Check sheet for the drawn part. Datum: minimum x, y, z corner. Units: mm. A direction names the side the tool comes from. Round coordinates to 2 decimals unless told otherwise and drop trailing zeros. Loops run counter-clockwise (first coordinate to the right, second up) from the corner with the lowest first, then second, coordinate; pieces in that order, holes last. Notation, with made-up numbers: (-26, -35.75) -> (10, -35.75) arc R4 cw to (10, -31.75) -> close; hole circle Ø1 at (43.25, 64.25). An arc over 180 degrees is marked (long way). Use CSV: the item, a comma, the result in double quotes. Start each with the question number.
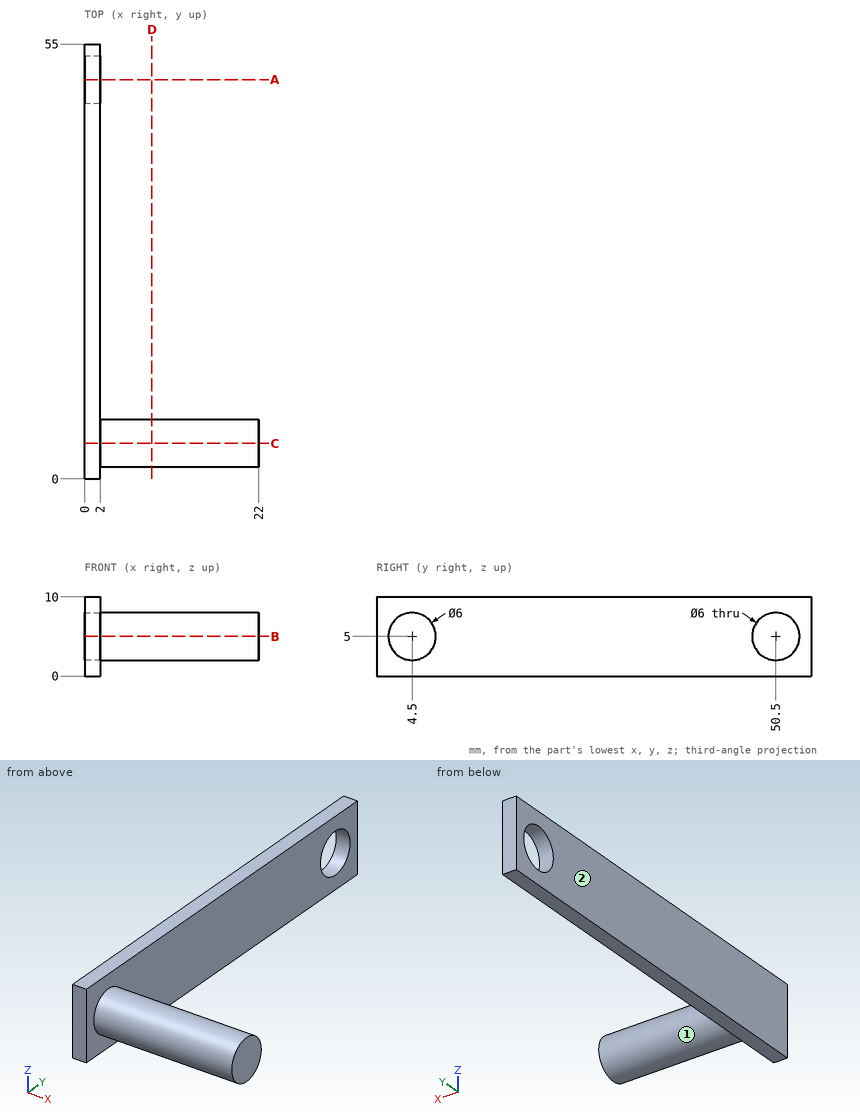
Q1. Cross-section at C-C (y = 4.5). Record the boundary of the cut face in (x, z), and give its area (3 significant figures).
Q2. Depth check by flat-ended pin: pin 1 Ø1 at (y, z) = (47, 6.5) entering from +X; pin 2 Ø4 at (y, z) = (27.5, 1.5) entering from -X; pin 3 Ø6 at (x, z) = (6, 3) entering from -Y. Enter the tip coordinate at first touch or a pass-through.
Q3. Tool access check on the marked faces 1 and 2. Record the directions out of +Z, -Z, +X, -X, +Y, -Y that give a thin tool (end or side, any length) a straight path to the whole face; none if there is none.
Q4. Cross-section at D-D (x = 8.5). Record the boundary of the cut face in (y, z), and give its area (3 significant figures).
Q5. Cross-section at B-B (z = 5). Record the boundary of the cut face in (x, y), and give its area (3 significant figures).
Q6. Thickness scan on L1, parallel to Y at x = 1.15, z = 5; L2, parallel to Y at x = 4.75, z = 4.75; L3, parallel to X at y = 36.5, z = 7. Record the ranges inside material, lowest first. Write a range as from..to.
Q7. Cross-section at A-A (y = 50.5). Record the boundary of the cut face in (x, z).
Answer list:
1,outline,"(0, 0) -> (2, 0) -> (2, 2) -> (22, 2) -> (22, 8) -> (2, 8) -> (2, 10) -> (0, 10) -> close"
1,area,"140 mm2"
2,pin 1,"stops at x = 2"
2,pin 2,"stops at x = 0"
2,pin 3,"stops at y = 1.5"
3,face 1,"+X"
3,face 2,"+Z, -Z, -X, +Y, -Y"
4,outline,"circle Ø6 at (4.5, 5)"
4,area,"28.3 mm2"
5,outline,"(0, 0) -> (2, 0) -> (2, 1.5) -> (22, 1.5) -> (22, 7.5) -> (2, 7.5) -> (2, 47.5) -> (0, 47.5) -> close; (0, 53.5) -> (2, 53.5) -> (2, 55) -> (0, 55) -> close"
5,area,"218 mm2"
6,L1,"y = 0..47.5, 53.5..55"
6,L2,"y = 1.51..7.49"
6,L3,"x = 0..2"
7,outline,"(0, 0) -> (2, 0) -> (2, 2) -> (0, 2) -> close; (0, 8) -> (2, 8) -> (2, 10) -> (0, 10) -> close"
